Build history of the part. All positions in model axes, mm. A direction names the side the tool comes from. Give positions to 0.01 mm unless a question says otherwise; leave off trailing zeros. Order: outer loops, then holes, each group sorted by start corner. A loop starts at its lowest first (then second) coordinate and runs counter-clockwise, first axis right, second up. Notation, with made-up numbers: (-39.75, 12) - (-1.75, 12) arc R5 cw to (-1.75, 16) - close; hole circle Ø8 at (-15, 0.5). An arc over 180 degrees is marked (long way). Answer in a Markdown table with one row per item.
```python
from build123d import *

# Parameters (mm, degrees)
SKETCH1_W           = 40
SKETCH1_H           = 40
SKETCH1_W_2         = 36
SKETCH1_H_2         = 36
EXTRUDE_THIN1_DEPTH = 350
FILLET1_R           = 0.5
FILLET2_R           = 2
SKETCH2_R           = 2.5
CUT_EXTRUDE1_DEPTH  = 352.140997322
CIRPATTERN1_COUNT   = 2
CIRPATTERN1_ANGLE   = 90


with BuildPart() as part:
    # Sketch1 → Extrude-Thin1 (new body)
    with BuildSketch(Plane.XY):
        Rectangle(SKETCH1_W, SKETCH1_H)
        Rectangle(SKETCH1_W_2, SKETCH1_H_2, mode=Mode.SUBTRACT)
    extrude(amount=EXTRUDE_THIN1_DEPTH)

    # Fillet1
    fillet1_edges = [part.edges().sort_by_distance(p)[0] for p in [
        (18, -18, 175),
        (18, 18, 175),
        (-18, 18, 175),
        (-18, -18, 175),
    ]]
    fillet(fillet1_edges, radius=FILLET1_R)

    # Fillet2
    fillet2_edges = [part.edges().sort_by_distance(p)[0] for p in [
        (20, -20, 175),
        (-20, -20, 175),
        (-20, 20, 175),
        (20, 20, 175),
    ]]
    fillet(fillet2_edges, radius=FILLET2_R)

    # Sketch2 → Cut-Extrude1 (cut, through all)
    with BuildSketch(Plane(origin=(0, 0, 0), x_dir=(0, 0, -1), z_dir=(1, 0, 0))):
        with Locations((-340, 0)):
            Circle(SKETCH2_R)
        with Locations((-315, 0)):
            Circle(SKETCH2_R)
    cut_extrude1 = extrude(amount=-CUT_EXTRUDE1_DEPTH, mode=Mode.SUBTRACT)

    # CirPattern1: Cut-Extrude1 ×2 about axis
    cirpattern1_axis = Axis((0, 0, 367.5), (0, 0, 1))
    for i in range(1, CIRPATTERN1_COUNT):
        add(cut_extrude1.rotate(cirpattern1_axis, i * CIRPATTERN1_ANGLE / (CIRPATTERN1_COUNT - 1)), mode=Mode.SUBTRACT)


solid = part.part
```
1. Probe line 1 (Z direction, x = 0, y = -19.55); line 2 (X direction, y = -1, z = 325.5). List the from-to ranges inside material, lowest first.
Check result:
| item | result |
|---|---|
| line 1 | z = 0 to 312.5, 317.5 to 337.5, 342.5 to 350 |
| line 2 | x = -20 to -18, 18 to 20 |
2. Two-plate mould, pull along Y, no slides. Class faces 3 (the face through (0, 20, 173)), 4 (the face through (0, -18, 173)), 5 (the face through (0, 19, 0)): +Y half, -Y half, draft (parallel to the pull), parting line (faces both ways), or undercut.
Check result:
| item | result |
|---|---|
| face 3 | +Y half |
| face 4 | undercut |
| face 5 | draft |
3. Drop a flat-ended pin along its axis: P1, Ø4.5, axis at y = 0, z = 315, coming from the -X side. Give the stop position or say it passes through.
Check result:
| item | result |
|---|---|
| P1 | stops at x = 18 |
4. Cut at A-A on z = 114. Write the cut outline in (x, y), and give its area (3 significant figures).
Check result:
| item | result |
|---|---|
| outline | (-20, -18) arc R2 ccw to (-18, -20) - (18, -20) arc R2 ccw to (20, -18) - (20, 18) arc R2 ccw to (18, 20) - (-18, 20) arc R2 ccw to (-20, 18) - close; hole (-18, -17.5) arc R0.5 ccw to (-17.5, -18) - (17.5, -18) arc R0.5 ccw to (18, -17.5) - (18, 17.5) arc R0.5 ccw to (17.5, 18) - (-17.5, 18) arc R0.5 ccw to (-18, 17.5) - close |
| area | 301 mm² |
5. Which spindle directions (+Z, -Z, +X, -X, +Y, -Y) get a long thin tool onto all of the face, cutting with end or side? Do faces 1 (the face through (-18, 0, 173)), 2 (the face through (-20, 0, 173)). Say none if no direction does.
Check result:
| item | result |
|---|---|
| face 1 | +Z, -Z |
| face 2 | +Z, -Z, -X, +Y, -Y |
6. Cut at B-B on y = -6. Write the cut outline in (x, z), and give its area (3 significant figures).
Check result:
| item | result |
|---|---|
| outline | (-20, 0) - (-18, 0) - (-18, 350) - (-20, 350) - close; (18, 0) - (20, 0) - (20, 350) - (18, 350) - close |
| area | 1,400 mm² |
